Model file for the job. Use its own axes, mm. Face numbers are marked on the shaded views. Round coordinates to 2 decimals unless told otherwise and drop trailing zeros. Loops run counter-clockwise (first coordinate to the right, second up) from the corner with the lowest first, then second, coordinate; pieces in that order, holes last. Notation, with made-up numbers: (38.5, 23) - (75.5, 23) arc R17 ccw to (75.5, 34) - close; hole circle Ø11 at (51, -31.75). An arc over 180 degrees is marked (long way). Answer as a JSON object with one key per item and string values.
from build123d import *

# Parameters (mm, degrees)
SKETCH_R     = 5
PAD_DEPTH    = 12
SKETCH001_R  = 27
PAD001_DEPTH = 28
SKETCH002_R  = 15
POCKET_DEPTH = 25


with BuildPart() as part:
    # Sketch → Pad (new body)
    with BuildSketch(Plane.XY):
        with BuildLine():
            ThreePointArc((7.2, 26.022298), (0, 27), (-7.2, 26.022298))
            Line((-49, 14.456832), (-7.2, 26.022298))
            ThreePointArc((-49, 14.456832), (-60, -1.6e-05), (-48.999969, -14.456841))
            Line((-7.2, -26.022298), (-48.999969, -14.456841))
            ThreePointArc((-7.2, -26.022298), (0, -27), (7.2, -26.022298))
            Line((49, -14.456832), (7.2, -26.022298))
            ThreePointArc((49, -14.456832), (60, 0), (49, 14.456832))
            Line((7.2, 26.022298), (49, 14.456832))
        make_face()
        with Locations((45, 0)):
            Circle(SKETCH_R, mode=Mode.SUBTRACT)
        with Locations((-45, 0)):
            Circle(SKETCH_R, mode=Mode.SUBTRACT)
    extrude(amount=PAD_DEPTH)

    # Sketch001 → Pad001 (new body)
    with BuildSketch(Plane.XY.offset(12)):
        Circle(SKETCH001_R)
    extrude(amount=PAD001_DEPTH)

    # Sketch002 → Pocket (cut)
    with BuildSketch(Plane.XY.offset(40)):
        Circle(SKETCH002_R)
    extrude(amount=-POCKET_DEPTH, mode=Mode.SUBTRACT)


solid = part.part
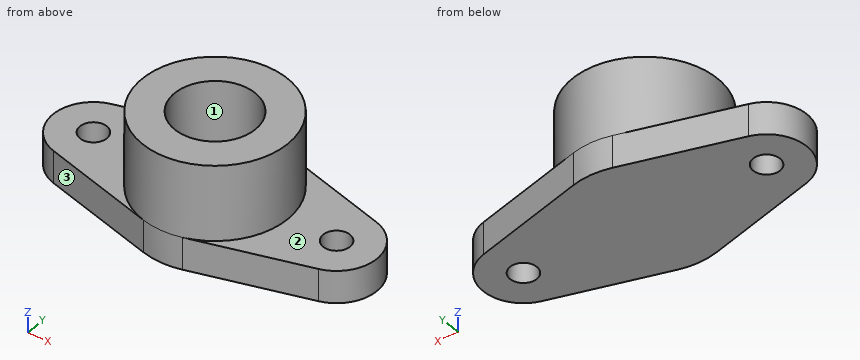
1) Two-plate mould, pull along X, no slides. Class the marked faces 1, 2 and 3: pulls with the +X half, pulls with the -X half, needs draft (parallel to the pull), parting line crosses it, or undercut.
Values follow:
{"face 1": "undercut", "face 2": "needs draft", "face 3": "pulls with the -X half"}
2) Slice it at D-D on x = -10. List the corners of the cut face in (y, z), then the cut area to 3 significant figures.
Values follow:
{"outline": "(-25.25, 0) - (25.25, 0) - (25.25, 12) - (25.08, 12) - (25.08, 40) - (11.18, 40) - (11.18, 15) - (-11.18, 15) - (-11.18, 40) - (-25.08, 40) - (-25.08, 12) - (-25.25, 12) - close", "area": "1,450 mm²"}
3) Drop flat-ended pins along their axis: P1, Ø5, axis at x = 6.5, z = 12.5, coming from the -Y side; P2, Ø2, axis at x = 1, z = 33, coming from the +Y side; P3, Ø2, axis at y = 13, z = 28, coming from the +X side. Give the stop position or say it passes through.
Values follow:
{"P1": "y = -26.7", "P2": "y = 27", "P3": "x = 24.19"}
4) Slice it at B-B on z = 3. List the corners of the cut face in (x, y), then the cut area to 4 significant figures.
Values follow:
{"outline": "(-49, -14.46) - (-7.2, -26.02) arc R27 ccw to (7.2, -26.02) - (49, -14.46) arc R15 ccw to (49, 14.46) - (7.2, 26.02) arc R27 ccw to (-7.2, 26.02) - (-49, 14.46) arc R15 ccw to start; hole circle Ø10 at (-45, 0); hole circle Ø10 at (45, 0)", "area": "4,465 mm²"}
5) Probe probe 1 along Y at (x, z) = (0, 21.25); probe 2 along Z at (x, y) = (-35, 4.5); probe 3 along Y at (x, z) = (45, 6). List the from-to ranges inside material, lowest first.
Values follow:
{"probe 1": "-27 to -15, 15 to 27", "probe 2": "0 to 12", "probe 3": "-15.56 to -5, 5 to 15.56"}
6) Slice it at A-A on y = 0. List the corners of the cut face in (x, z).
Values follow:
{"outline": "(-60, 0) - (-50, 0) - (-50, 12) - (-60, 12) - close; (-40, 0) - (40, 0) - (40, 12) - (27, 12) - (27, 40) - (15, 40) - (15, 15) - (-15, 15) - (-15, 40) - (-27, 40) - (-27, 12) - (-40, 12) - close; (50, 0) - (60, 0) - (60, 12) - (50, 12) - close"}
7) Slice it at C-C on x = 45. List the corners of the cut face in (y, z).
Values follow:
{"outline": "(-15.56, 0) - (-5, 0) - (-5, 12) - (-15.56, 12) - close; (5, 0) - (15.56, 0) - (15.56, 12) - (5, 12) - close"}
